from build123d import *

# Parameters (mm, degrees)
SKETCH1_W           = 122.2
SKETCH1_H           = 65.54
BOSS_EXTRUDE1_DEPTH = 3
SKETCH2_W           = 80
SKETCH2_H           = 2
BOSS_EXTRUDE2_DEPTH = 10
FILLET1_R           = 1
SKETCH3_W           = 80
SKETCH3_H           = 2
CUT_EXTRUDE1_DEPTH  = 7
SKETCH4_W           = 80
SKETCH4_H           = 2.5
BOSS_EXTRUDE3_DEPTH = 3
FILLET2_R           = 1
CUT_EXTRUDE2_DEPTH  = 10
CUT_EXTRUDE3_DEPTH  = 10
SKETCH7_W           = 122.2
SKETCH7_H           = 3
BOSS_EXTRUDE4_DEPTH = 6
SKETCH8_R           = 1
CUT_EXTRUDE4_DEPTH  = 6
FILLET3_R           = 2


with BuildPart() as part:
    # Sketch1 → Boss-Extrude1 (new body)
    with BuildSketch(Plane(origin=(0, 0, 0), x_dir=(1, 0, 0), z_dir=(0, 1, 0))):
        Rectangle(SKETCH1_W, SKETCH1_H)
    extrude(amount=BOSS_EXTRUDE1_DEPTH)

    # Sketch2 → Boss-Extrude2 (add)
    with BuildSketch(Plane(origin=(0, 3, 0), x_dir=(1, 0, 0), z_dir=(0, 1, 0))):
        with Locations((0, -9.73)):
            Rectangle(SKETCH2_W, SKETCH2_H)
        with Locations((0, -14.43)):
            Rectangle(SKETCH2_W, SKETCH2_H)
    extrude(amount=BOSS_EXTRUDE2_DEPTH)

    # Fillet1
    fillet1_edges = [part.edges().sort_by_distance(p)[0] for p in [
        (40, 3, 14.43),
        (0, 3, 15.43),
        (-40, 3, 14.43),
        (40, 3, 9.73),
        (0, 3, 8.73),
        (-40, 3, 9.73),
    ]]
    fillet(fillet1_edges, radius=FILLET1_R)

    # Sketch3 → Cut-Extrude1 (cut)
    with BuildSketch(Plane(origin=(0, 13, 0), x_dir=(1, 0, 0), z_dir=(0, 1, 0))):
        with Locations((0, -9.73)):
            Rectangle(SKETCH3_W, SKETCH3_H)
        with Locations((0, -14.43)):
            Rectangle(SKETCH3_W, SKETCH3_H)
    extrude(amount=-CUT_EXTRUDE1_DEPTH, mode=Mode.SUBTRACT)

    # Sketch4 → Boss-Extrude3 (add)
    with BuildSketch(Plane(origin=(0, 3, 0), x_dir=(1, 0, 0), z_dir=(0, 1, 0))):
        with Locations((0, -29.02)):
            Rectangle(SKETCH4_W, SKETCH4_H)
    boss_extrude3 = extrude(amount=BOSS_EXTRUDE3_DEPTH)

    # Fillet2
    fillet2_edges = [part.edges().sort_by_distance(p)[0] for p in [
        (40, 3, 29.02),
        (0, 3, 27.77),
        (-40, 3, 29.02),
    ]]
    fillet(fillet2_edges, radius=FILLET2_R)

    # Mirror1: Boss-Extrude3 across plane
    add(boss_extrude3.mirror(Plane.ZY))

    # Sketch5 → Cut-Extrude2 (cut)
    with BuildSketch(Plane(origin=(0, 3, 0), x_dir=(1, 0, 0), z_dir=(0, 1, 0))):
        with BuildLine():
            Line((48.1, 22.77), (6.311514948, 22.77))
            Line((6.311514948, 22.77), (-48.1, 22.77))
            ThreePointArc((-48.1, 22.77), (-50.221320344, 21.891320344), (-51.1, 19.77))
            Line((-51.1, 19.77), (-51.1, 3.77))
            ThreePointArc((-51.1, 3.77), (-50.221320344, 1.648679656), (-48.1, 0.77))
            Line((-48.1, 0.77), (48.1, 0.77))
            ThreePointArc((48.1, 0.77), (50.221320344, 1.648679656), (51.1, 3.77))
            Line((51.1, 3.77), (51.1, 19.77))
            ThreePointArc((51.1, 19.77), (50.221320344, 21.891320344), (48.1, 22.77))
        make_face()
    extrude(amount=-CUT_EXTRUDE2_DEPTH, mode=Mode.SUBTRACT)

    # Sketch6 → Cut-Extrude3 (cut)
    with BuildSketch(Plane(origin=(0, 3, 0), x_dir=(1, 0, 0), z_dir=(0, 1, 0))):
        with BuildLine():
            ThreePointArc((24.574193631, -24.893622011), (23.513533459, -24.454282183), (23.074193631, -23.393622011))
            Line((23.074193631, -23.393622011), (23.074193631, -18.473462095))
            ThreePointArc((23.074193631, -18.473462095), (23.659980069, -17.059248532), (25.074193631, -16.473462095))
            Line((25.074193631, -16.473462095), (38.784700518, -16.473462095))
            Line((38.784700518, -16.473462095), (44.284700518, -16.473462095))
            Line((44.284700518, -16.473462095), (44.284700518, -5.054704437))
            ThreePointArc((44.284700518, -5.054704437), (44.964391332, -3.856403354), (46.257750275, -3.381927082))
            Line((46.257750275, -3.381927082), (50.626867349, -3.381927082))
            ThreePointArc((50.626867349, -3.381927082), (51.392234214, -3.534168016), (52.041080911, -3.967713519))
            Line((52.041080911, -3.967713519), (55.687864116, -7.614496724))
            ThreePointArc((55.687864116, -7.614496724), (55.921387017, -7.895147518), (56.1, -8.213573672))
            Line((56.1, -8.213573672), (56.1, -21.269749634))
            ThreePointArc((56.1, -21.269749634), (55.074873734, -23.744623369), (52.6, -24.769749634))
            Line((52.6, -24.769749634), (46.32782558, -24.769749634))
            Line((46.32782558, -24.769749634), (39.284700518, -24.893622011))
            Line((39.284700518, -24.893622011), (24.574193631, -24.893622011))
        make_face()
        with BuildLine():
            ThreePointArc((20.660852384, -23.893622011), (20.367959165, -24.600728792), (19.660852384, -24.893622011))
            Line((19.660852384, -24.893622011), (4.043952302, -24.893622011))
            ThreePointArc((4.043952302, -24.893622011), (3.336845521, -24.600728792), (3.043952302, -23.893622011))
            Line((3.043952302, -23.893622011), (3.043952302, -19.096324264))
            ThreePointArc((3.043952302, -19.096324264), (3.48329213, -18.035664092), (4.543952302, -17.596324264))
            Line((4.543952302, -17.596324264), (19.160852384, -17.596324264))
            ThreePointArc((19.160852384, -17.596324264), (20.221512556, -18.035664092), (20.660852384, -19.096324264))
            Line((20.660852384, -19.096324264), (20.660852384, -23.893622011))
        make_face()
        with BuildLine():
            ThreePointArc((-20.660852384, -19.096324264), (-20.221512556, -18.035664092), (-19.160852384, -17.596324264))
            Line((-19.160852384, -17.596324264), (-4.543952302, -17.596324264))
            ThreePointArc((-4.543952302, -17.596324264), (-3.48329213, -18.035664092), (-3.043952302, -19.096324264))
            Line((-3.043952302, -19.096324264), (-3.043952302, -23.893622011))
            ThreePointArc((-3.043952302, -23.893622011), (-3.336845521, -24.600728792), (-4.043952302, -24.893622011))
            Line((-4.043952302, -24.893622011), (-19.660852384, -24.893622011))
            ThreePointArc((-19.660852384, -24.893622011), (-20.367959165, -24.600728792), (-20.660852384, -23.893622011))
            Line((-20.660852384, -23.893622011), (-20.660852384, -19.096324264))
        make_face()
        with BuildLine():
            Line((-56.1, -21.269749634), (-56.1, -8.213573672))
            ThreePointArc((-56.1, -8.213573672), (-55.921387017, -7.895147518), (-55.687864116, -7.614496724))
            Line((-55.687864116, -7.614496724), (-52.041080911, -3.967713519))
            ThreePointArc((-52.041080911, -3.967713519), (-51.392234214, -3.534168016), (-50.626867349, -3.381927082))
            Line((-50.626867349, -3.381927082), (-46.257750275, -3.381927082))
            ThreePointArc((-46.257750275, -3.381927082), (-44.964391332, -3.856403354), (-44.284700518, -5.054704437))
            Line((-44.284700518, -5.054704437), (-44.284700518, -22.726624573))
            ThreePointArc((-44.284700518, -22.726624573), (-44.883117994, -24.171332159), (-46.32782558, -24.769749634))
            Line((-46.32782558, -24.769749634), (-52.6, -24.769749634))
            ThreePointArc((-52.6, -24.769749634), (-55.074873734, -23.744623369), (-56.1, -21.269749634))
        make_face()
        with BuildLine():
            Line((-39.284700518, -24.893622011), (-24.574193631, -24.893622011))
            ThreePointArc((-24.574193631, -24.893622011), (-23.513533459, -24.454282183), (-23.074193631, -23.393622011))
            Line((-23.074193631, -23.393622011), (-23.074193631, -18.473462095))
            ThreePointArc((-23.074193631, -18.473462095), (-23.659980069, -17.059248532), (-25.074193631, -16.473462095))
            Line((-25.074193631, -16.473462095), (-38.784700518, -16.473462095))
            ThreePointArc((-38.784700518, -16.473462095), (-40.198914081, -17.059248532), (-40.784700518, -18.473462095))
            Line((-40.784700518, -18.473462095), (-40.784700518, -23.393622011))
            ThreePointArc((-40.784700518, -23.393622011), (-40.34536069, -24.454282183), (-39.284700518, -24.893622011))
        make_face()
    extrude(amount=-CUT_EXTRUDE3_DEPTH, mode=Mode.SUBTRACT)

    # Sketch7 → Boss-Extrude4 (add)
    with BuildSketch(Plane.XY.offset(32.77)):
        with Locations((0, 1.5)):
            Rectangle(SKETCH7_W, SKETCH7_H)
    extrude(amount=BOSS_EXTRUDE4_DEPTH)

    # Sketch8 → Cut-Extrude4 (cut)
    with BuildSketch(Plane.XZ):
        with Locations((0, 35.77)):
            Circle(SKETCH8_R)
        with Locations((-27.15, 35.77)):
            Circle(SKETCH8_R)
        with Locations((27.15, 35.77)):
            Circle(SKETCH8_R)
    extrude(amount=-CUT_EXTRUDE4_DEPTH, mode=Mode.SUBTRACT)

    # Fillet3
    fillet3_edges = [part.edges().sort_by_distance(p)[0] for p in [
        (44.284700518, 1.5, 16.473462095),
    ]]
    fillet(fillet3_edges, radius=FILLET3_R)


solid = part.part
For this review, take the finished solid that the model builds, in its own axes (mm). A direction names the side the tool comes from. Give positions to 0.01 mm unless a question says otherwise; leave off trailing zeros. Order: outer loops, then holes, each group sorted by start corner. A loop starts at its lowest first (then second) coordinate and runs counter-clockwise, first axis right, second up. Notation, with made-up numbers: (26, 79) -> (82, 79) arc R30 cw to (82, 116) -> close; hole circle Ø11 at (38.5, 76). An arc over 180 degrees is marked (long way). Write item = value, one per line.
1) We need section A-A, the plane y = 5. Give the boundary of the cut face in (x, z).
Findings:
outline = (-40, 8.73) -> (40, 8.73) -> (40, 10.73) -> (-40, 10.73) -> close; (-40, 13.43) -> (40, 13.43) -> (40, 15.43) -> (-40, 15.43) -> close; (-40, 27.77) -> (40, 27.77) -> (40, 30.27) -> (-40, 30.27) -> close
2) Insertion check: pin 1 (1.6 mm diameter, centred on y = 5.5, z = 14.5, fed in from -X); pin 2 (1.6 mm diameter, centred on y = 5, z = 28.5, fed in from +X). Each pin has a flat end and moves straight along its axis. Give the tip position at first contact, or say it passes through.
Findings:
pin_1 = -40
pin_2 = 40
3) We need section B-B, the plane z = -8. Give the boundary of the cut face in (x, y).
Findings:
outline = (-61.1, 0) -> (-51.1, 0) -> (-51.1, 3) -> (-61.1, 3) -> close; (51.1, 0) -> (61.1, 0) -> (61.1, 3) -> (51.1, 3) -> close
4) We need section C-C, the plane z = -28. Give the boundary of the cut face in (x, y), and give its area (3 significant figures).
Findings:
outline = (-61.1, 0) -> (61.1, 0) -> (61.1, 3) -> (-61.1, 3) -> close
area = 367 mm^2
5) To check wall thickness, follow L1, parallel to Z at x = 0, y = 1.3; L2, parallel to Z at x = 27.15, y = 1.15; L3, parallel to Z at x = 34, y = 4.4. State the ranges of each line that lie inside material, in increasing order. Write a range as from..to.
Findings:
L1 = -32.77..-22.77, -0.77..34.77, 36.77..38.77
L2 = -32.77..-22.77, -0.77..16.47, 24.89..34.77, 36.77..38.77
L3 = 8.73..10.73, 13.43..15.43, 27.77..30.27
6) For faces 4 (the face through (-12, 2, 24.894)), 5 (the face through (-1, 4, 30.27)), 6 (the face through (-1, 6, 29)), list the 3-axis set-ups (+Z, -Z, +X, -X, +Y, -Y) from which the entire face can be reached by the end or side of a thin tool; tool diameter is ignored.
Findings:
face_4 = +Y, -Y
face_5 = +Z, +X, -X, +Y
face_6 = +Z, -Z, +X, -X, +Y
7) Draft analysis for pull direction X (two halves, no side actions). For faces 1 (the face through (-23.074, 2, 21)), 2 (the face through (-1, 4, 10.73)), 3 (the face through (61.1, 1, 2)), state which applies: pulls with the +X half, pulls with the -X half, needs draft (parallel to the pull), parting line crosses it, or undercut.
Findings:
face_1 = undercut
face_2 = needs draft
face_3 = pulls with the +X half
